from build123d import *

# Parameters (mm, degrees)
EXTRU_MINCE1_DEPTH    = 55
D_GAGEMENT_M41_D      = 4.5
D_GAGEMENT_M42_D      = 4.5
D_GAGEMENT_M271_D     = 30
D_GAGEMENT_M271_DEPTH = 1.5
D_GAGEMENT_M271_TIP   = 9.012909285


with BuildPart() as part:
    # Esquisse1 → Extru.-Mince1 (new body)
    with BuildSketch(Plane.XY):
        Polygon((0, 39), (0, 0), (25, 0), (25, 1.5), (1.5, 1.5), (1.5, 39), align=None)
    extrude(amount=-EXTRU_MINCE1_DEPTH)

    # Dégagement M41 (through all)
    with Locations(Plane(origin=(0, 1.5, 0), x_dir=(-1, 0, 0), z_dir=(0, 1, 0))):
        with Locations((-12.5, -7), (-12.5, -27.5), (-12.5, -48)):
            Hole(D_GAGEMENT_M41_D / 2)

    # Dégagement M42 (through all)
    with Locations(Plane(origin=(1.5, 0, 0), x_dir=(0, 0, -1), z_dir=(1, 0, 0))):
        with Locations((6, 33.5), (34, 5.5)):
            Hole(D_GAGEMENT_M42_D / 2)

    # Dégagement M271
    with Locations(Plane(origin=(1.5, 0, 0), x_dir=(0, 0, -1), z_dir=(1, 0, 0))):
        with Locations((20, 19.5)):
            Hole(D_GAGEMENT_M271_D / 2, depth=D_GAGEMENT_M271_DEPTH)
            with Locations((0, 0, -(D_GAGEMENT_M271_DEPTH + D_GAGEMENT_M271_TIP / 2))):  # 118° drill point
                Cone(0, D_GAGEMENT_M271_D / 2, D_GAGEMENT_M271_TIP, mode=Mode.SUBTRACT)


solid = part.part
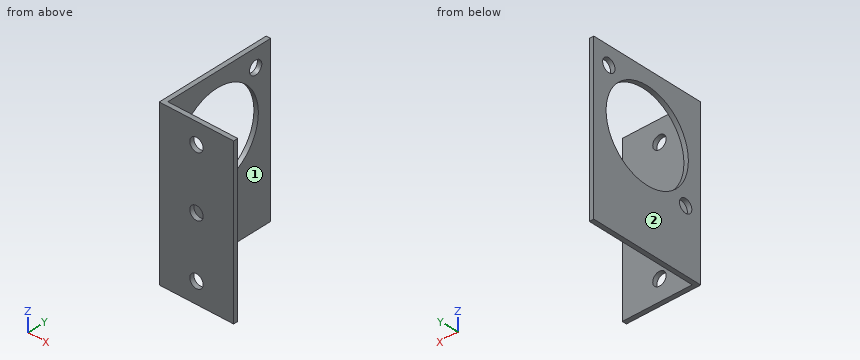
Verification items for the finished model (mm, model axes). Face numbers are marked on the shaded views. A direction names the side the tool comes from. Give positions to 0.01 mm unless a question says otherwise; leave off trailing zeros. Loops run counter-clockwise (first coordinate to the right, second up) from the corner with the lowest first, then second, coordinate; pieces in that order, holes last. Notation, with made-up numbers: (44, 57) - (98, 57) arc R16 ccw to (98, 66) - close; hole circle Ø10 at (-30.75, -39). An arc over 180 degrees is marked (long way). Write each question's results on one line, items separated by ' | '.
1) Sectioned sample at A-A on z = -20. Record the boundary of the cut face in (x, y).
Solution:
outline: (0, 0) - (25, 0) - (25, 1.5) - (1.5, 1.5) - (1.5, 4.5) - (0, 4.5) - close; (0, 34.5) - (1.5, 34.5) - (1.5, 39) - (0, 39) - close
2) Material ranges on L1, parallel to Y at x = 0.5, z = -20; L2, parallel to X at y = 37.5, z = -23, recorded low to high. Write a range as from..to.
Solution:
L1: 0..4.5, 34.5..39 | L2: 0..1.5
3) Sectioned sample at D-D on y = 21. Record the boundary of the cut face in (x, z).
Solution:
outline: (0, -55) - (1.5, -55) - (1.5, -34.92) - (0, -34.92) - close; (0, -5.08) - (1.5, -5.08) - (1.5, 0) - (0, 0) - close
4) Depth check by flat-ended pin: P1, Ø3.5, axis at x = 12.5, z = -48, coming from the +Y side (1 decimal); P2, Ø10, axis at x = 8.5, z = -40.5, coming from the +Y side; P3, Ø12, axis at y = 16, z = -33.5, coming from the +X side. Enter the tip coordinate at first touch or a pass-through.
Solution:
P1: through | P2: y = 1.5 | P3: x = 1.5
5) Tool access check on the marked faces 1 and 2. Record the directions out of +Z, -Z, +X, -X, +Y, -Y that give a thin tool (end or side, any length) a straight path to the whole face; none if there is none.
Solution:
face 1: +Z, -Z, +X, +Y | face 2: +Z, -Z, -X, +Y, -Y
6) Sectioned sample at B-B on x = 12.5. Record the boundary of the cut face in (y, z).
Solution:
outline: (0, -55) - (1.5, -55) - (1.5, -50.25) - (0, -50.25) - close; (0, -45.75) - (1.5, -45.75) - (1.5, -29.75) - (0, -29.75) - close; (0, -25.25) - (1.5, -25.25) - (1.5, -9.25) - (0, -9.25) - close; (0, -4.75) - (1.5, -4.75) - (1.5, 0) - (0, 0) - close
7) Sectioned sample at C-C on y = 33.5. Record the boundary of the cut face in (x, z).
Solution:
outline: (0, -55) - (1.5, -55) - (1.5, -25.39) - (0, -25.39) - close; (0, -14.61) - (1.5, -14.61) - (1.5, -8.25) - (0, -8.25) - close; (0, -3.75) - (1.5, -3.75) - (1.5, 0) - (0, 0) - close
